Could you check a few things on this drawing? It's one solid part, dimensions in mm from its lowest x, y, z. A direction names the side the tool comes from. Give positions to 0.01 mm unless a question says otherwise; leave off trailing zeros. Loops run counter-clockwise (first coordinate to the right, second up) from the corner with the lowest first, then second, coordinate; pieces in that order, holes last. Notation, with made-up numbers: (-13, 41.5) - (2, 41.5) arc R12 cw to (2, 52.5) - close; hole circle Ø1 at (-17, 49). An arc over 180 degrees is marked (long way). Answer as a JSON object with one key per item and string values.
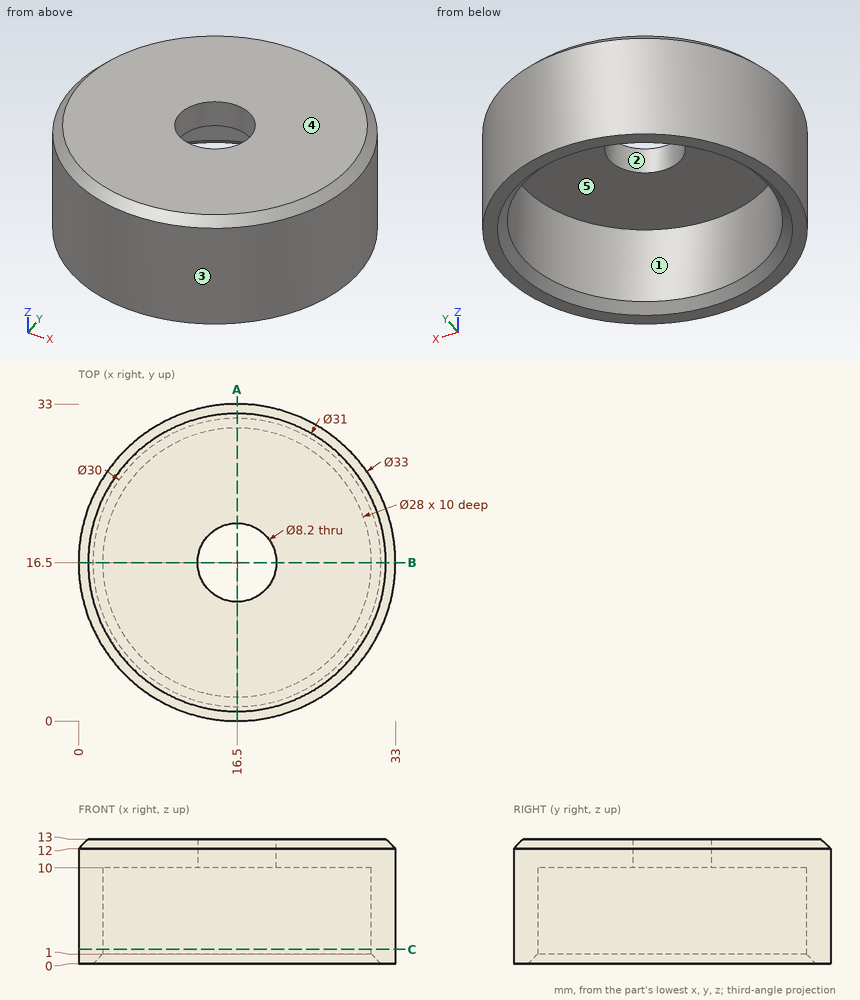
1) Imagine slicing it at A-A on x = 16.5. Write out the boundary of the cut face in (y, z).
Check sheet entries:
{"outline": "(0, 0) - (1.5, 0) - (2.5, 1) - (2.5, 10) - (12.4, 10) - (12.4, 13) - (1, 13) - (0, 12) - close; (20.6, 10) - (30.5, 10) - (30.5, 1) - (31.5, 0) - (33, 0) - (33, 12) - (32, 13) - (20.6, 13) - close"}
2) If we mould it in two halves opening along Y, with no side actions, what happens to the marked faces 3, 4 and 5? For each: released by +Y, released by -Y, zero draft, split by the parting line, or undercut.
Check sheet entries:
{"face 3": "split by the parting line", "face 4": "zero draft", "face 5": "undercut"}
3) I'm going to push flat-ended pins straight in: P1, Ø1, axis at x = 12.5, z = 10, coming from the +Y side; P2, Ø2, axis at x = 10, y = 23.5, coming from the -Z side; P3, Ø3, axis at x = 6, z = 6, coming from the +Y side; P4, Ø4, axis at x = 15.5, z = 9, coming from the +Y side. Where does each tip first touch, or does it pass through?
Check sheet entries:
{"P1": "y = 32.62", "P2": "z = 10", "P3": "y = 30.33", "P4": "y = 33"}
4) Which directions (+Z, -Z, +X, -X, +Y, -Y) give clear straight access to the entire face, cutting with the end or side of a thin tool? Please do the marked faces 1 and 2.
Check sheet entries:
{"face 1": "-Z", "face 2": "+Z, -Z"}
5) I need wall thicknesses on L1, parallel to Y at x = 16.5, z = 5.5; L2, parallel to Y at x = 16.5, z = 11.5; L3, parallel to Z at x = 22, y = 13. Which ranges of each line are inside material? Lowest first, please.
Check sheet entries:
{"L1": "0 to 2.5, 30.5 to 33", "L2": "0 to 12.4, 20.6 to 33", "L3": "10 to 13"}
6) Imagine slicing it at C-C on z = 1.5. Write out the boundary of the cut face in (x, y), and give its area (3 significant figures).
Check sheet entries:
{"outline": "circle Ø33 at (16.5, 16.5); hole circle Ø28 at (16.5, 16.5)", "area": "240 mm2"}
